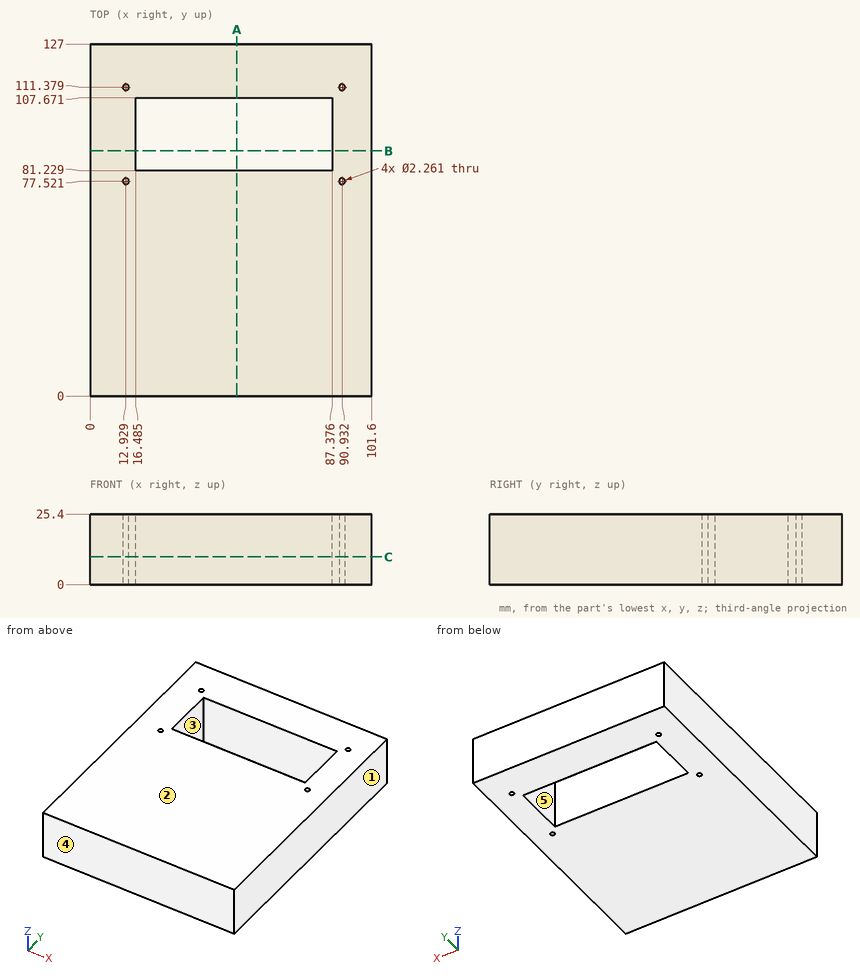
Input: dimensioned drawing with shaded views. Units: mm. Origin: part minimum x, y, z. A direction names the side the tool comes from. Coordinates: 2 decimals unless noted, no trailing zeros. Loops run counter-clockwise (first coordinate to the right, second up) from the corner with the lowest first, then second, coordinate; pieces in that order, holes last. Notation, with made-up numbers: (-16, 84) - (34, 84) arc R16 ccw to (34, 113) - close; hole circle Ø2 at (75, 31.5). An arc over 180 degrees is marked (long way). One line per question, with ' | ' between items. Start each with the question number.
(1) First-contact query: pin 1 (1 mm diameter, centred on x = 76.5, z = 15.5, fed in from -Y). Flat tip, straight axial feed; report the tip coordinate or a pass-through.
(2) Cut plane C-C on z = 10. Output: boundary loops of the cut face in (x, y) (1 decimal).
(3) Draft query along X for the marked faces 1, 2 and 3. Return one class per face: +X half, -X half, draft (parallel to the pull), parting line (faces both ways), or undercut.
(4) Cut plane A-A on x = 53. Output: boundary loops of the cut face in (y, z), and give its area (3 significant figures).
(5) Cut plane B-B on y = 88.5. Output: boundary loops of the cut face in (x, z) (1 decimal), and give its area (3 significant figures).
(6) Ray query, L1, parallel to Y at x = 65, z = 11.25; L2, parallel to X at y = 100, z = 12.25 (1 decimal). Return the intervals inside material, ascending. Write a range as from..to.
(7) Reachability of the marked faces 4 and 5 from +Z, -Z, +X, -X, +Y, -Y: full face, straight path, thin tool, end or side. Return the list, or none.
Here are the results:
1) pin 1: y = 0
2) outline: (0, 0) - (101.6, 0) - (101.6, 127) - (0, 127) - close; hole circle Ø2.3 at (12.9, 77.5); hole circle Ø2.3 at (12.9, 111.4); hole (16.5, 81.2) - (87.4, 81.2) - (87.4, 107.7) - (16.5, 107.7) - close; hole circle Ø2.3 at (90.9, 77.5); hole circle Ø2.3 at (90.9, 111.4)
3) face 1: +X half | face 2: draft | face 3: undercut
4) outline: (0, 0) - (81.23, 0) - (81.23, 25.4) - (0, 25.4) - close; (107.67, 0) - (127, 0) - (127, 25.4) - (107.67, 25.4) - close | area: 2,550 mm²
5) outline: (0, 0) - (16.5, 0) - (16.5, 25.4) - (0, 25.4) - close; (87.4, 0) - (101.6, 0) - (101.6, 25.4) - (87.4, 25.4) - close | area: 780 mm²
6) L1: 0..81.23, 107.67..127 | L2: 0..16.5, 87.4..101.6
7) face 4: +Z, -Z, +X, -X, -Y | face 5: +Z, -Z
